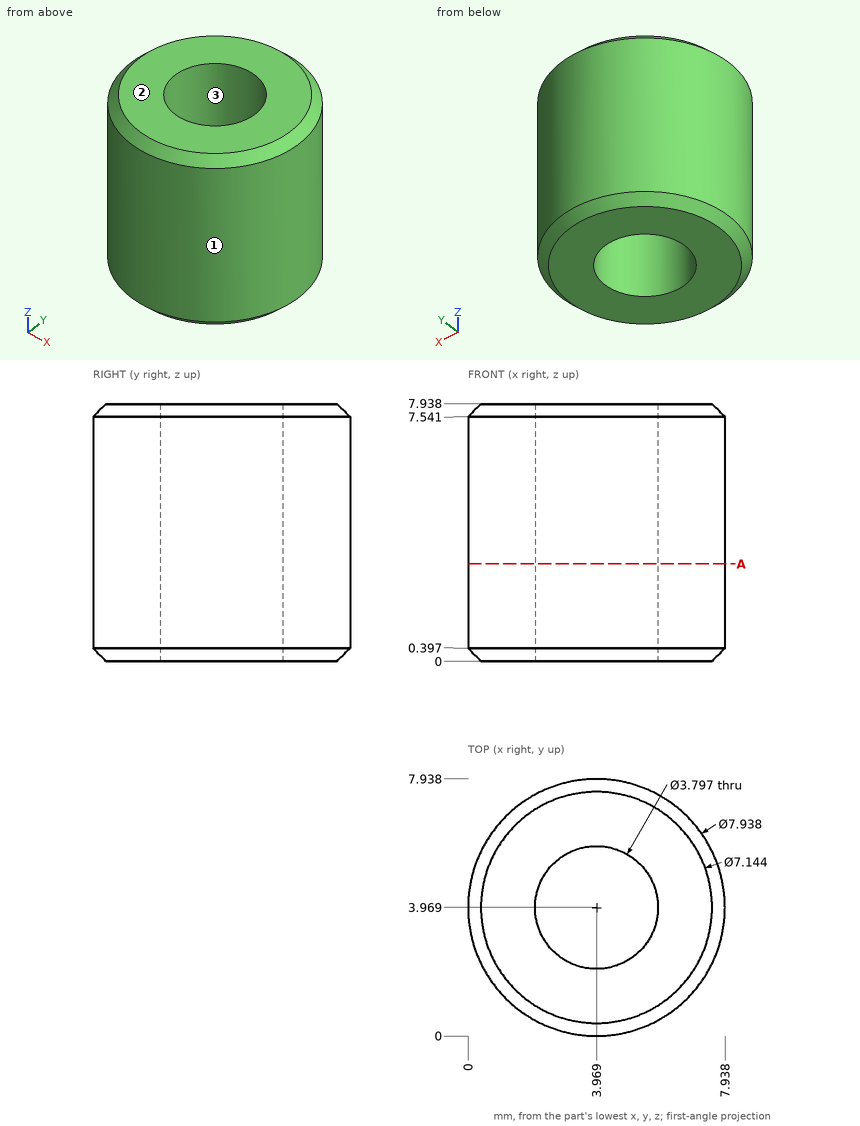
Design review of the part shown in the three views and the two pictorial views. Dimensions are in mm from the part's minimum x, y and z. Give positions to 0.01 mm unless a question says otherwise; leave off trailing zeros. Loops run counter-clockwise (first coordinate to the right, second up) from the corner with the lowest first, then second, coordinate; pieces in that order, holes last. Notation, with made-up numbers: M 11.5,71.5 L 56.5,71.5 A20 ccw 56.5,92.5 Z; hole C 1,-21.5 d9. An arc over 180 degrees is marked long. Put each result on its own line as item: value. Start each with the question number.
(1) The part is to be moulded in two halves that separate along Y. For the marked faces 1, 2 and 3, say which applies: +Y half, -Y half, draft (parallel to the pull), parting line (faces both ways), or undercut.
(2) For pin 1 (3 mm diameter, centred on y = 6.5, z = 2.5, fed in from -X), flat-tipped, find the tip position at first contact; note if it passes through.
(3) Wall thickness on L1, parallel to Y at x = 4, z = 2; L2, parallel to X at y = 3.25, z = 3 (1 decimal); L3, parallel to X at y = 3.5, z = 2: over which ranges is each line inside the solid? List them lowest first.
(4) Add section A-A, the plane z = 3. Write out the cut boundary in (x, y).
Result:
1. face 1: parting line
1. face 2: draft
1. face 3: undercut
2. pin 1: stops at x = 0.14
3. L1: y = 0 to 2.07, 5.87 to 7.94
3. L2: x = 0.1 to 2.2, 5.7 to 7.9
3. L3: x = 0.03 to 2.13, 5.81 to 7.91
4. outline: C 3.97,3.97 d7.94; hole C 3.97,3.97 d3.8
